from build123d import *

# Parameters (mm, degrees)
SALIENTE_EXTRUIR1_DEPTH = 500
REDONDEO1_R             = 2
REDONDEO2_R             = 2
REDONDEO4_R             = 0.5


with BuildPart() as part:
    # Croquis1 → Saliente-Extruir1 (new body)
    with BuildSketch(Plane.XY):
        Polygon((-4.451940983, 8.315120378), (1.548059017, 8.315120378), (1.548059017, 13.315120378), (5.548059017, 13.315120378), (5.548059017, -6.684879622), (1.548059017, -6.684879622), (1.548059017, -1.684879622), (-4.451940983, -1.684879622), (-4.451940983, -32.384879622), (5.548059017, -32.384879622), (5.548059017, -28.384879622), (1.548059017, -28.384879622), (1.548059017, -23.250181803), (19.548059017, -23.250181803), (19.548059017, -28.384879622), (15.548059017, -28.384879622), (15.548059017, -32.384879622), (25.548059017, -32.384879622), (25.548059017, -1.684879622), (19.548059017, -1.684879622), (19.548059017, -6.684879622), (15.548059017, -6.684879622), (15.548059017, 13.315120378), (19.548059017, 13.315120378), (19.548059017, 8.315120378), (25.548059017, 8.315120378), (25.548059017, 35.015120378), (1.548059017, 35.015120378), (1.548059017, 45.015120378), (-4.451940983, 45.015120378), align=None)
    extrude(amount=SALIENTE_EXTRUIR1_DEPTH)

    # Redondeo1
    redondeo1_edges = [part.edges().sort_by_distance(p)[0] for p in [
        (25.548059017, -32.384879622, 250),
        (-4.451940983, -32.384879622, 250),
    ]]
    fillet(redondeo1_edges, radius=REDONDEO1_R)

    # Redondeo2
    redondeo2_edges = [part.edges().sort_by_distance(p)[0] for p in [
        (19.548059017, -28.384879622, 250),
        (1.548059017, -28.384879622, 250),
    ]]
    fillet(redondeo2_edges, radius=REDONDEO2_R)

    # Redondeo4
    redondeo4_edges = [part.edges().sort_by_distance(p)[0] for p in [
        (19.548059017, -1.684879622, 250),
        (25.548059017, -1.684879622, 250),
        (15.548059017, -32.384879622, 250),
        (15.548059017, -28.384879622, 250),
        (5.548059017, -28.384879622, 250),
        (5.548059017, -32.384879622, 250),
        (-4.451940983, -1.684879622, 250),
        (1.548059017, -1.684879622, 250),
        (1.548059017, 8.315120378, 250),
        (-4.451940983, 8.315120378, 250),
        (-4.451940983, 45.015120378, 250),
        (1.548059017, 45.015120378, 250),
        (25.548059017, 35.015120378, 250),
        (25.548059017, 8.315120378, 250),
        (19.548059017, 8.315120378, 250),
    ]]
    fillet(redondeo4_edges, radius=REDONDEO4_R)


solid = part.part
Can you work these out from the model? Positions are in its coordinate system, mm. A direction names the side the tool comes from. Coordinates: 2 decimals unless noted, no trailing zeros. Write item = value, one per line.
(1) For pin 1 (7 mm diameter, centred on x = 8.5, z = 223, fed in from +Y); pin 2 (12 mm diameter, centred on y = -1, z = 141, fed in from +X); pin 3 (1 mm diameter, centred on x = 19.5, y = 7, fed in from -Z); pin 4 (1 mm diameter, centred on x = 15.5, z = 50, fed in from -Y), each with a flat end and sliding along its axis, tell me the tip position at first contact or that it passes through.
Verdict:
pin_1 = 35.02
pin_2 = 25.55
pin_3 = through
pin_4 = -32.38
(2) Thinking about a two-plate mould opening in Y: for faces 4 (the face through (-4.452, -16, 246)), 5 (the face through (13, 35.015, 246)), 6 (the face through (15.548, 3, 246)), which applies, +Y half, -Y half, draft (parallel to the pull), parting line (faces both ways), or undercut?
Verdict:
face_4 = draft
face_5 = +Y half
face_6 = undercut
(3) If I drill on probe 1 along Y at (x, z) = (16.25, 20); probe 2 along Y at (x, z) = (5.25, 403.5); probe 3 along X at (y, z) = (-6.5, 367), over which ranges is the centre line in solid material (lowest first)?
Verdict:
probe_1 = -32.38 to -28.38, -23.25 to -6.68, 13.32 to 35.02
probe_2 = -32.34 to -28.43, -23.25 to -6.68, 13.32 to 35.02
probe_3 = -4.45 to 1.55, 5.55 to 15.55, 19.55 to 25.55
(4) On a 3-axis mill with a long thin cutter (end or side, diameter ignored), from which of +Z, -Z, +X, -X, +Y, -Y can I reach the whole of each face in a straight line? I mean faces 1 (the face through (1.548, 40, 246)), 2 (the face through (25.548, 21, 246)), 3 (the face through (5.548, 3, 246)). Say none if no direction works.
Verdict:
face_1 = +Z, -Z, +X, +Y
face_2 = +Z, -Z, +X, +Y, -Y
face_3 = +Z, -Z
